from build123d import *

# Parameters (mm, degrees)
PAD_DEPTH       = 34.25
SKETCH001_R     = 1.25
POCKET_DEPTH    = 10
SKETCH002_W     = 70.5
SKETCH002_H     = 12.89
PAD001_DEPTH    = 3
SKETCH003_W     = 15
SKETCH003_H     = 2.8
POCKET001_DEPTH = 37.251
SKETCH004_W     = 5
SKETCH004_H     = 3.5
POCKET002_DEPTH = 37.251
SKETCH005_R     = 1.5
POCKET003_DEPTH = 37.251
SKETCH006_R     = 0.5
POCKET004_DEPTH = 37.251
CHAMFER_SIZE    = 0.5


with BuildPart() as part:
    # Sketch → Pad (new body)
    with BuildSketch(Plane.XY):
        with BuildLine():
            Line((52.305921, 0), (60.5, 0))
            ThreePointArc((60.5, 0), (63.426078, 3.661869), (59.208881, 5.707953))
            Line((59.208881, 5.707953), (48.64775, 0.672534))
            ThreePointArc((48.64775, 0.672534), (47.930845, 0.287572), (47.254036, -0.164179))
            ThreePointArc((39.665197, 0.854908), (43.253158, -1.19207), (47.254036, -0.164179))
            ThreePointArc((39.665197, 0.854908), (32.988877, 4.094039), (26.312556, 0.854908))
            ThreePointArc((17.672613, 0.854908), (21.992584, -1.241), (26.312556, 0.854908))
            ThreePointArc((17.672613, 0.854908), (10.996292, 4.094039), (4.319972, 0.854908))
            ThreePointArc((0, -1.241), (2.400781, -0.689359), (4.319972, 0.854908))
            Line((0, -2.741), (0, -1.241))
            ThreePointArc((0, -2.741), (3.055539, -2.038911), (5.498146, -0.073481))
            ThreePointArc((16.494438, -0.073481), (10.996292, 2.594039), (5.498146, -0.073481))
            ThreePointArc((16.494438, -0.073481), (21.992584, -2.741), (27.490731, -0.073481))
            ThreePointArc((38.487023, -0.073481), (32.988877, 2.594039), (27.490731, -0.073481))
            ThreePointArc((38.487023, -0.073481), (43.053519, -2.678725), (48.145545, -1.3705))
            ThreePointArc((52.305921, 0), (50.115773, -0.351448), (48.145545, -1.3705))
        make_face()
    extrude(amount=PAD_DEPTH)

    # Sketch001 (on Face17 of Pad) → Pocket (cut)
    with BuildSketch(Plane(origin=(0, 0, 0), x_dir=(1, 0, 0), z_dir=(0, 0, -1))):
        with Locations((60.5, -3)):
            Circle(SKETCH001_R)
    extrude(amount=-POCKET_DEPTH, mode=Mode.SUBTRACT)

    # Sketch002 (on Face5 of Pocket) → Pad001 (join)
    with BuildSketch(Plane.XY.offset(34.25)):
        with Locations((35.25, 1.145)):
            Rectangle(SKETCH002_W, SKETCH002_H)
    extrude(amount=PAD001_DEPTH)

    # Sketch003 (on Face23 of Pad001) → Pocket001 (cut, through all)
    with BuildSketch(Plane.XY.offset(37.25)):
        with Locations((63, -3.9)):
            Rectangle(SKETCH003_W, SKETCH003_H)
    extrude(amount=-POCKET001_DEPTH, mode=Mode.SUBTRACT)

    # Sketch004 (on Face25 of Pocket001) → Pocket002 (cut, through all)
    with BuildSketch(Plane.XY.offset(37.25)):
        with Locations((68, 5.84)):
            Rectangle(SKETCH004_W, SKETCH004_H)
    extrude(amount=-POCKET002_DEPTH, mode=Mode.SUBTRACT)

    # Sketch005 (on Face27 of Pocket002) → Pocket003 (cut, through all)
    with BuildSketch(Plane.XY.offset(37.25)):
        with Locations((68, 1)):
            Circle(SKETCH005_R)
    extrude(amount=-POCKET003_DEPTH, mode=Mode.SUBTRACT)

    # Sketch006 (on Face28 of Pocket003) → Pocket004 (cut, through all)
    with BuildSketch(Plane.XY.offset(37.25)):
        with Locations((65.5, 4.09)):
            Circle(SKETCH006_R)
        with Locations((55.5, -2.5)):
            Circle(SKETCH006_R)
    extrude(amount=-POCKET004_DEPTH, mode=Mode.SUBTRACT)

    # Chamfer
    chamfer_edges = [part.edges().sort_by_distance(p)[0] for p in [
        (70.5, 4.09, 35.75),
        (70.5, -2.5, 35.75),
    ]]
    chamfer(chamfer_edges, length=CHAMFER_SIZE)

    # Mirrored: part across YZ


with BuildPart() as part_1:
    add(part.part)
    add(part.part.mirror(Plane.YZ))


solid = part_1.part
Could you check a few things on this model? Use its own coordinates, in mm. A direction names the side the tool comes from. Give positions to 0.01 mm unless a question says otherwise; leave off trailing zeros. Loops run counter-clockwise (first coordinate to the right, second up) from the corner with the lowest first, then second, coordinate; pieces in that order, holes last. Notation, with made-up numbers: (80, 81) -> (111, 81) arc R13 ccw to (111, 106) -> close; hole circle Ø4 at (16.5, 23). An arc over 180 degrees is marked (long way). Answer as CSV lines item,"result". Start each with the question number.
(1) We'd pull the mould along Y, two halves only. Please class faces 4 (the cylindrical face through (21.92, -1.24, 16.89)), 5 (the cylindrical face through (69.43, 1.45, 35.77)), 6 (the flat face through (1, 1, 37.25)): released by +Y, released by -Y, zero draft, split by the parting line, or undercut.
(2) If we section it at B-B on x = 24: Write out the boundary of the cut face in (y, z), then the cut area to 3 significant figures.
(3) I'm going to push flat-ended pins straight in: pin 1 Ø2.5 at (x, z) = (63.5, 36) entering from -Y; pin 2 Ø1.5 at (x, z) = (67.5, 35) entering from +Y; pin 3 Ø0.7 at (y, z) = (-3.5, 35.5) entering from -X; pin 4 Ø2.5 at (x, y) = (68, 1) entering from +Z. Where does each tip first touch, or does it pass through?
(4) I need wall thicknesses on probe 1 along Y at (x, z) = (-68, 35); probe 2 along Y at (x, z) = (-60.5, 6); probe 3 along Z at (x, y) = (48, 5.75). Which ranges of each line are inside material? Lowest first, please.
(5) Which directions (+Z, -Z, +X, -X, +Y, -Y) give clear straight access to the entire face, cutting with the end or side of a thin tool? Please do faces 1 (the flat face through (-65.5, 6, 36)), 2 (the flat face through (-55.5, -4, 36)), 3 (the flat face through (60, 3, 10)).
Computed:
1,face 4,"released by +Y"
1,face 5,"undercut"
1,face 6,"zero draft"
2,outline,"(-5.3, 34.25) -> (-2.45, 34.25) -> (-2.45, 0) -> (-0.86, 0) -> (-0.86, 34.25) -> (7.59, 34.25) -> (7.59, 37.25) -> (-5.3, 37.25) -> close"
2,area,"93.0 mm2"
3,pin 1,"stops at y = -2.5"
3,pin 2,"stops at y = 4.09"
3,pin 3,"stops at x = -55.5"
3,pin 4,"passes through"
4,probe 1,"y = -2.5 to -0.5, 2.5 to 4.09"
4,probe 2,"y = 0 to 1.75, 4.25 to 6"
4,probe 3,"z = 34.25 to 37.25"
5,face 1,"+Z, -Z, -X, +Y"
5,face 2,"+Z, -Z, -X, -Y"
5,face 3,"-Z"
